Autodesk Inventor part; units mm, degrees
ref_plane "YZ Plane" through (0, 0, 0) normal (1, 0, 0) x (0, 1, 0)
ref_plane "XZ Plane" through (0, 0, 0) normal (0, 1, 0) x (-1, 0, 0)
ref_plane "XY Plane" through (0, 0, 0) normal (0, 0, 1) x (1, 0, 0)
sketch "Sketch1" plane through (0, 0, 0) normal (0, 0, 1) x (1, 0, 0)
  line L0 (0, 0) -> (114.3, 0)
  line L1 (0, 0) -> (0, -50.8)
  line L2 (0, -50.8) -> (114.3, -50.8)
  line L3 (114.3, -50.8) -> (114.3, 0)
  dimension "d1" = 114.3
  dimension "d2" = 50.8
  dimension "d3" = 114.3
extrude "Extrusion1" add sketch "Sketch1" along normal blind 3.175
sketch "Sketch2" plane through (0, 0, 0) normal (0, 1, 0) x (1, 0, 0)
  line L0 (114.3, -3.175) -> (0, -3.175)
  line L1 (25.3873, -1.5875) -> (25.3873, 0)
  line L2 (25.3873, -3.175) -> (25.3873, -1.5875)
  line L3 (28.7401, -1.5875) -> (28.7401, -3.175)
  line L4 (28.7401, -1.5875) -> (28.7401, 0)
  line L5 (25.3873, -3.175) -> (22.2123, -3.175)
  line L6 (22.2123, -3.175) -> (22.2123, 3.175)
  line L7 (28.7401, -3.175) -> (31.9151, -3.175)
  line L8 (31.9151, -3.175) -> (31.9151, 3.175)
  line L9 (25.3873, 0) -> (25.3873, 3.175)
  line L10 (25.3873, 3.175) -> (22.2123, 3.175)
  line L11 (31.9151, 3.175) -> (28.7401, 3.175)
  line L12 (28.7401, 3.175) -> (28.7401, 0)
  point P0 (27.0637, -1.5875)
  dimension "d7" = 1.6764
  dimension "d8" = 1.6764
  dimension "d9" = 3.175
  dimension "d10" = 6.35
  dimension "d11" = 3.175
sketch "Sketch3" plane through (0, 0, 0) normal (0, 0, -1) x (-1, 0, 0)
  line L0 (-114.3, 0) -> (0, 0)
  line L1 (0, -50.8) -> (-114.3, -50.8)
  line L2 (0, 0) -> (-114.3, 0)
  line L3 (-114.3, 0) -> (-114.3, -50.8)
  line L4 (-114.3, -50.8) -> (0, -50.8)
  line L5 (0, -50.8) -> (0, 0)
extrude "Extrusion2" add sketch "Sketch3" along normal blind 3.175
extrude "Extrusion3" add sketch "Sketch2" along normal blind 76.2 contours L0 L3 L4 L12 L11 L8
extrude "Extrusion4" add sketch "Sketch2" along normal blind 76.2 contours L0 L6 L10 L9 L1 L2
sketch "Sketch4" plane through (31.9151, 0, 3.175) normal (1, 0, 0) x (0, 0, -1)
  line L0 (3.175, 0) -> (3.175, 19.05)
  circle A0 centre (3.175, 19.05) radius 1.5875
  dimension "d18" = 19.05
  dimension "d19" = 3.175
extrude "Extrusion5" cut sketch "Sketch4" along normal mid plane 50.8
sketch "Sketch5" plane through (31.9151, 0, 3.175) normal (1, 0, 0) x (0, 0, -1)
  circle A0 centre (3.175, 19.05) radius 1.5875
  line L0 (3.175, 19.05) -> (3.175, 60.706)
  circle A1 centre (3.175, 60.706) radius 1.5875
  point P0 (3.175, 0)
  dimension "d22" = 41.656
  dimension "d23" = 3.175
extrude "Extrusion6" cut sketch "Sketch5" against normal blind 50.8 contours A1
sketch "Sketch6" plane through (25.3873, 0, 3.175) normal (1, 0, 0) x (0, 0, -1)
  point P0 (3.175, 0)
sketch "Sketch7" plane through (0, 0, 3.175) normal (0, 0, 1) x (1, 0, 0)
  point P0 (0, 0)
sketch "Sketch8" plane through (0, 0, 3.175) normal (0, 0, 1) x (1, 0, 0)
  line L0 (38.0873, 0) -> (41.2623, 0)
  line L1 (41.2623, 0) -> (41.2623, 22.5425)
  line L2 (38.0873, 0) -> (38.0873, 22.5425)
  line L3 (38.0873, 22.5425) -> (41.2623, 22.5425)
  line L4 (38.0873, 22.5425) -> (31.9151, 22.5425)
  line L5 (31.9151, 0) -> (31.9151, 76.2)
  line L6 (41.2623, 22.5425) -> (41.2623, 25.7175)
  line L7 (41.2623, 25.7175) -> (31.9151, 25.7175)
  point P0 (0, 0)
  dimension "d30" = 3.175
  dimension "d34" = 3.175
sketch "Sketch9" plane through (0, 0, 3.175) normal (0, 0, 1) x (1, 0, 0)
  line L0 (41.2623, 25.7175) -> (41.2623, 0)
  line L1 (31.9151, 0) -> (114.3, 0)
  line L2 (44.6151, 0) -> (44.6151, 25.6324)
  line L3 (44.6151, 25.6324) -> (47.7901, 25.6324)
  line L4 (47.7901, 0) -> (47.7901, 25.6324)
  line L5 (44.6151, 0) -> (47.7901, 0)
  point P0 (0, 0)
  dimension "d35" = 3.3528
  dimension "d36" = 3.175
sketch "Sketch12" plane through (0, 0, 3.175) normal (0, 0, 1) x (1, 0, 0)
  line L0 (44.6151, 0) -> (44.6151, 25.6324)
  line L1 (44.6151, 0) -> (46.3169, 0)
  line L2 (46.3169, 0) -> (49.4919, 0)
  line L3 (25.3873, 0) -> (114.3, 0)
  line L4 (49.4919, 0) -> (49.4919, 25.6324)
  line L5 (49.4919, 25.6324) -> (46.3169, 25.6324)
  line L6 (46.3169, 25.6324) -> (46.3169, 0)
  point P0 (0, 0)
  point P1 (47.7901, 0)
  point P2 (41.2623, 0)
  dimension "d44" = 1.7018
  dimension "d45" = 3.175
extrude "Extrusion11" add sketch "Sketch12" against normal blind 6.35
sketch "Sketch13" plane through (0, 0, 3.175) normal (0, 0, 1) x (1, 0, 0)
  line L0 (38.0873, 22.5425) -> (38.0873, 0)
  line L1 (38.0873, 0) -> (39.7891, 0)
  line L2 (39.7891, 0) -> (42.9641, 0)
  line L3 (46.3169, 0) -> (31.9151, 0)
  line L4 (39.7891, 0) -> (39.7891, 25.7175)
  line L5 (41.2623, 25.7175) -> (31.9151, 25.7175)
  line L6 (42.9641, 0) -> (42.9641, 25.7175)
  line L7 (42.9641, 25.7175) -> (39.7891, 25.7175)
  point P0 (0, 0)
  point P1 (41.2623, 0)
  dimension "d48" = 1.7018
  dimension "d49" = 3.175
extrude "Extrusion12" add sketch "Sketch13" against normal blind 6.35
sketch "Sketch14" plane through (0, 0, 3.175) normal (0, 0, 1) x (1, 0, 0)
  line L0 (39.7891, 25.7175) -> (42.9641, 25.7175)
  line L1 (39.7891, 25.7175) -> (39.7891, 22.5425)
  line L2 (39.7891, 25.7175) -> (39.7891, 0)
  line L3 (39.7891, 22.5425) -> (31.9151, 22.5425)
  line L4 (39.7891, 25.7175) -> (50.9246, 25.7175) construction
  line L5 (42.9641, 25.7175) -> (56.7757, 25.7175) construction
  line L6 (31.9151, 0) -> (31.9151, 76.2)
  line L7 (31.9151, 36.7665) -> (42.9641, 25.7175)
  line L8 (31.9151, 36.7665) -> (31.9151, 22.5425)
  line L9 (42.9641, 25.7175) -> (39.7891, 25.7175)
  line L10 (39.7891, 25.7175) -> (42.9641, 25.7175)
  point P0 (0, 0)
  dimension "d52" = 3.175
extrude "Extrusion13" add sketch "Sketch14" against normal blind 6.35
sketch "Sketch15" plane through (22.2123, 0, -3.175) normal (-1, 0, 0) x (0, 0, 1)
  circle A0 centre (3.175, 19.05) radius 1.5875
  circle A1 centre (3.175, 19.05) radius 1.5875
  point P0 (3.175, 0)
extrude "Extrusion14" cut sketch "Sketch15" against normal blind 50.8
sketch "Sketch16" plane through (0, 0, 3.175) normal (0, 0, 1) x (1, 0, 0)
  line L0 (31.9151, 36.7665) -> (42.9641, 25.7175)
  line L1 (42.9641, 25.7175) -> (22.2123, 25.7175)
  line L2 (22.2123, 0) -> (22.2123, 76.2)
  line L3 (42.9641, 25.7175) -> (42.9641, 0)
  line L4 (42.9641, 0) -> (22.2123, 0)
  line L5 (22.2123, 0) -> (22.2123, 25.7175)
  line L6 (42.9641, 25.7175) -> (42.9641, 0)
  point P0 (0, 0)
extrude "Extrusion15" add sketch "Sketch16" against normal blind 6.35
sketch "Sketch17" plane through (49.4919, 0, 3.175) normal (1, 0, 0) x (0, 0, -1)
  circle A0 centre (3.175, 19.05) radius 1.5875
  circle A1 centre (3.175, 19.05) radius 1.5875
  point P0 (3.175, 0)
extrude "Extrusion16" cut sketch "Sketch17" against normal blind 12.7
fillet "Fillet1" radius 1.5875 2 edges at (42.9641, 0, 0) (46.3169, 0, 0)
fillet "Fillet2" radius 1.5875 8 edges at (25.3873, 25.7175, 0) (28.7401, 25.7175, 0) (22.2123, 0, 0) (0, 0, 0) (49.4919, 0, 0) (114.3, 0, 0) (114.3, -50.8, 0) (0, -50.8, 0)
fillet "Fillet3" radius 1.5875 1 edges at (31.9151, 36.7665, 0)
properties part number "2BarClawPaddle" material "Aluminum 6061"
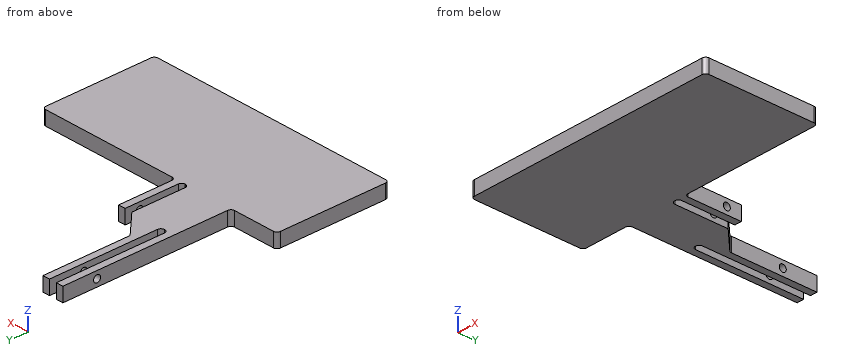
Source: CAD feature listing. Evaluate the final solid. Frame: model axes, mm. Give positions to 0.01 mm unless a question says otherwise; leave off trailing zeros. Order: outer loops, then holes, each group sorted by start corner. A loop starts at its lowest first (then second) coordinate and runs counter-clockwise, first axis right, second up.
(1) Section query B-B (z = 0). State how many separate pieces and enclosed holes the cut face has, plus the area to 3 significant figures.
(2) Section query A-A (y = 13.5). Return the cut outline in (x, z) (3 decimals).
(3) Material intervals for line 1 along Y through (x, z) = (30.65, 0); line 2 along Y through (x, z) = (48.15, 0); line 3 along X through (y, z) = (7.5, -3), sorted ascending.
(4) Section query D-D (y = 33.5). Return the cut outline in (x, z) (3 decimals).
(5) Contact query for flat-ended pins moving along their axis: P1, Ø2.5, axis at y = 19.05, z = 0, coming from the +X side; P2, Ø1.9, axis at y = 17.5, z = -0.5, coming from the -X side; P3, Ø1.9, axis at y = 61, z = -1.5, coming from the +X side. Output: stop coordinate, or through.
Outcome:
1. separate pieces: 4
1. enclosed holes: 0
1. area: 6,750 mm2
2. outline: (22.212, -3.175) - (42.964, -3.175) - (42.964, 3.175) - (22.212, 3.175) - close; (46.317, -3.175) - (49.492, -3.175) - (49.492, 3.175) - (46.317, 3.175) - close
3. line 1: y = -50.8 to 59.12, 62.29 to 76.2
3. line 2: y = -50.8 to 17.46, 20.64 to 25.63
3. line 3: x = 22.21 to 42.96, 46.32 to 49.49
4. outline: (22.212, -3.175) - (25.387, -3.175) - (25.387, 3.175) - (22.212, 3.175) - close; (28.74, -3.175) - (35.182, -3.175) - (35.182, 3.175) - (28.74, 3.175) - close
5. P1: stops at x = 36.79
5. P2: stops at x = 22.21
5. P3: stops at x = 31.92
